Here's the drawing with two shaded views (mm, measured from the low corner). I have some questions. A direction names the side the tool comes from. Coordinates: 2 decimals unless noted, no trailing zeros. Write each loop counter-clockwise with the first axis right and the second up, starting at its lowest first coordinate (ties: lowest second). Pieces come first, ordered by that corner, then holes. Notation, with made-up numbers: M 29.25,29 L 86.25,29 A28 cw 86.25,66 Z; hole C 14.5,17.5 d8. An arc over 180 degrees is marked long. Use one line per item in the form item = value. Start each with the question number.
1. I want a section at A-A, the plane x = 19. List the corners of the cut face in (y, z) for me, plus the area to 3 significant figures.
2. I want a section at C-C, the plane z = 30.5. List the corners of the cut face in (x, y) for me, plus the area to 3 significant figures.
3. I want a section at D-D, the plane x = 14.3. List the corners of the cut face in (y, z) for me.
4. I'm going to push flat-ended pins straight in: pin 1 Ø2.5 at (x, y) = (11, 15) entering from +Z; pin 2 Ø1 at (x, z) = (5, 35) entering from +Y; pin 3 Ø3.5 at (x, z) = (20, 39) entering from -Y. Where does each tip first touch, or does it pass through?
5. I want a section at B-B, the plane y = 8. List the corners of the cut face in (x, z) for me, plus the area to 3 significant figures.
6. Please list where these lines run through material, in increasing order: line 1 along Z through (x, y) = (7, 2.25); line 2 along Z through (x, y) = (25.25, 8.25); line 3 along X through (y, z) = (6, 5.5). Write a range as [from, to].
7. On a 3-axis mill with a long thin cutter (end or side, diameter ignored), from which of +Z, -Z, +X, -X, +Y, -Y can I reach the whole of each face in a straight line? I mean the marked faces 1, 2, 3 and 4. Say none if no direction works.
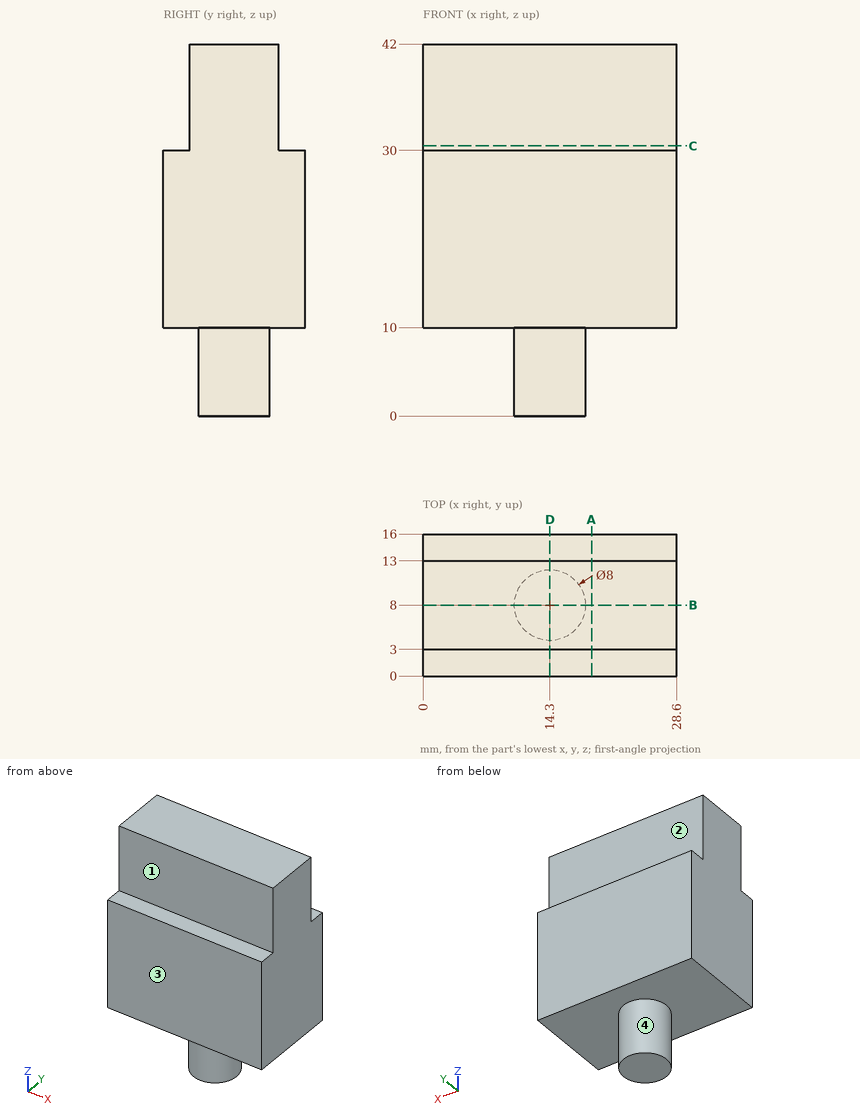
Answer list:
q1.outline = M 0,10 L 16,10 L 16,30 L 13,30 L 13,42 L 3,42 L 3,30 L 0,30 Z
q1.area = 440 mm²
q2.outline = M 0,3 L 28.6,3 L 28.6,13 L 0,13 Z
q2.area = 286 mm²
q3.outline = M 0,10 L 4,10 L 4,0 L 12,0 L 12,10 L 16,10 L 16,30 L 13,30 L 13,42 L 3,42 L 3,30 L 0,30 Z
q4.pin_1 = 30
q4.pin_2 = 13
q4.pin_3 = 3
q5.outline = M 0,10 L 10.3,10 L 10.3,0 L 18.3,0 L 18.3,10 L 28.6,10 L 28.6,42 L 0,42 Z
q5.area = 995 mm²
q6.line_1 = [10, 30]
q6.line_2 = [10, 42]
q6.line_3 = [10.84, 17.76]
q7.face_1 = +Z, +X, -X, -Y
q7.face_2 = +Z, +X, -X, +Y
q7.face_3 = +Z, -Z, +X, -X, -Y
q7.face_4 = -Z
